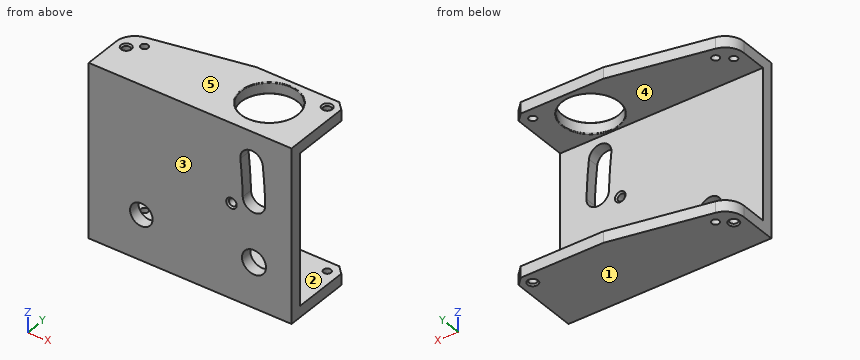
from build123d import *

# Parameters (mm, degrees)
SKETCH1_W      = 27
SKETCH1_H      = 23
SKETCH1_R      = 1.6
SKETCH1_R_2    = 1.5
SKETCH1_R_3    = 0.5
EXTRUDE1_DEPTH = 1.5
SKETCH2_R      = 0.5
SKETCH2_R_2    = 3.75
EXTRUDE2_DEPTH = 1.5
SKETCH3_R      = 0.5
EXTRUDE3_DEPTH = 1.5
FILLET1_R      = 0.1
CHAMFER1_SIZE  = 0.2
FILLET2_R      = 2.5


with BuildPart() as part:
    # Sketch1 → Extrude1 (new body)
    with BuildSketch(Plane(origin=(0, 0, 0), x_dir=(1, 0, 0), z_dir=(0, 1, 0))):
        with Locations((-8.5, -5.5)):
            Rectangle(SKETCH1_W, SKETCH1_H)
        with Locations(Location((0, 0, 0), (0, 0, 270))):  # turned: the seam where the file's is
            Circle(SKETCH1_R, mode=Mode.SUBTRACT)
        with Locations(Location((-15, 0, 0), (0, 0, 270))):  # turned: the seam where the file's is
            Circle(SKETCH1_R_2, mode=Mode.SUBTRACT)
        with Locations(Location((-3, -6.5, 0), (0, 0, 270))):  # turned: the seam where the file's is
            Circle(SKETCH1_R_3, mode=Mode.SUBTRACT)
        with BuildLine():
            ThreePointArc((-1.814657257, -12.850061187), (-1.613249333, -10.406431255), (-1.49938813, -7.957160339))
            ThreePointArc((-1.49938813, -7.957160339), (0.042839661, -6.50061187), (1.49938813, -8.042839661))
            ThreePointArc((1.49938813, -8.042839661), (1.380542383, -10.599333203), (1.170317351, -13.149938813))
            ThreePointArc((1.170317351, -13.149938813), (-0.472108766, -14.492487304), (-1.814657257, -12.850061187))
        make_face(mode=Mode.SUBTRACT)
    extrude(amount=EXTRUDE1_DEPTH)

    # Sketch2 → Extrude2 (add)
    with BuildSketch(Plane.XY.offset(17)):
        Polygon((-22, 1.5), (5, 1.5), (5, 9), (4, 10), (-7, 10), (-22, 7), align=None)
        with Locations((3.5, 8.5)):
            Circle(SKETCH2_R, mode=Mode.SUBTRACT)
        with Locations((-2, 5.5)):
            Circle(SKETCH2_R_2, mode=Mode.SUBTRACT)
        with Locations((-20.5, 4.75)):
            Circle(SKETCH2_R, mode=Mode.SUBTRACT)
        with Locations((-19, 6)):
            Circle(SKETCH2_R, mode=Mode.SUBTRACT)
    extrude(amount=-EXTRUDE2_DEPTH)

    # Sketch3 → Extrude3 (add)
    with BuildSketch(Plane(origin=(0, 0, -6), x_dir=(-1, 0, 0), z_dir=(0, 0, -1))):
        Polygon((-5, 1.5), (22, 1.5), (22, 7), (7, 10), (-4, 10), (-5, 9), align=None)
        with Locations(Location((-3.5, 8.5, 0), (0, 0, 180))):  # turned: the seam where the file's is
            Circle(SKETCH3_R, mode=Mode.SUBTRACT)
        with Locations(Location((20.5, 4.75, 0), (0, 0, 180))):  # turned: the seam where the file's is
            Circle(SKETCH3_R, mode=Mode.SUBTRACT)
        with Locations(Location((19, 6, 0), (0, 0, 180))):  # turned: the seam where the file's is
            Circle(SKETCH3_R, mode=Mode.SUBTRACT)
    extrude(amount=-EXTRUDE3_DEPTH)

    # Fillet1
    fillet1_edges = [part.edges().sort_by_distance(p)[0] for p in [
        (-5.75, 5.5, 15.5),
        (-5.75, 5.5, 17),
    ]]
    fillet(fillet1_edges, radius=FILLET1_R)

    # Chamfer1
    chamfer1_edges = [part.edges().sort_by_distance(p)[0] for p in [
        (-3, 0, 6),
        (-3, 1.5, 6),
        (3, 8.5, 17),
        (-21, 4.75, 17),
        (3, 8.5, -6),
        (-21, 4.75, -6),
    ]]
    chamfer(chamfer1_edges, length=CHAMFER1_SIZE)

    # Fillet2
    fillet2_edges = [part.edges().sort_by_distance(p)[0] for p in [
        (-22, 7, 16.25),
        (-22, 7, -5.25),
    ]]
    fillet(fillet2_edges, radius=FILLET2_R)


solid = part.part
Read the model definition and answer for the solid it produces. Units are mm, in the model's axes. Face numbers are marked on the shaded views. A direction names the side the tool comes from. Round coordinates to 2 decimals unless told otherwise and drop trailing zeros. Order: outer loops, then holes, each group sorted by start corner. A loop starts at its lowest first (then second) coordinate and runs counter-clockwise, first axis right, second up. Notation, with made-up numbers: (67.5, 12.25) - (104.5, 12.25) arc R29 ccw to (104.5, 47.25) - close; hole circle Ø6 at (48.5, 6.25). An arc over 180 degrees is marked (long way). Use one line per item in the form item = value. Start each with the question number.
(1) The part is cut by section D-D (x = 0). Count the separate pieces of the cut face and the enclosed holes in it, then the cut area to 3 significant figures.
(2) The part is cut by section C-C (z = 4). Give the vertices of the cut face in (x, y), then the cut area to 3 significant figures.
(3) The part is cut by section A-A (x = -19). Give the vertices of the cut face in (y, z).
(4) The part is cut by section B-B (z = 9). Give the vertices of the cut face in (x, y).
(5) Determine the mould class of the marked faces 3, 4 and 5 for opening direction Z: +Z half, -Z half, draft (parallel to the pull), parting line (faces both ways), or undercut.
(6) For the marked faces 1 and 2, determine the directions among +Z, -Z, +X, -X, +Y, -Y from which every point of the face is accessible in a straight line to the end or side of a thin tool.
(7) Find the intervals of material crossed by line 1 along Z through (x, y) = (-7.25, 3); line 2 along X through (y, z) = (0.9, 0); line 3 along Y through (x, z) = (-18.75, 12.25), in increasing order. Write a range as from..to.
(8) Flat-ended cylindrical pins translate along their axes: pin 1 Ø8 at (x, z) = (-9, -1) entering from +Y; pin 2 Ø1.5 at (x, z) = (-8, 3) entering from +Y; pin 3 Ø4.5 at (x, y) = (-2, 5.5) entering from +Z. Find the tip coordinate at first contact, or state that the pin passes through.
Checked values:
q1.separate_pieces = 4
q1.enclosed_holes = 0
q1.area = 33.7 mm^2
q2.outline = (-22, 0) - (5, 0) - (5, 1.5) - (-22, 1.5) - close
q2.area = 40.5 mm^2
q3.outline = (0, -6) - (5.5, -6) - (5.5, -4.5) - (1.5, -4.5) - (1.5, 15.5) - (5.5, 15.5) - (5.5, 17) - (0, 17) - close; (6.5, -6) - (7.6, -6) - (7.6, -4.5) - (6.5, -4.5) - close; (6.5, 15.5) - (7.6, 15.5) - (7.6, 17) - (6.5, 17) - close
q4.outline = (-22, 0) - (-1.54, 0) - (-1.54, 1.5) - (-22, 1.5) - close; (1.47, 0) - (5, 0) - (5, 1.5) - (1.47, 1.5) - close
q5.face_3 = draft
q5.face_4 = undercut
q5.face_5 = +Z half
q6.face_1 = -Z, +X, -X, +Y, -Y
q6.face_2 = +X, -X, +Y
q7.line_1 = -6..-4.5, 15.5..17
q7.line_2 = -22..-16.5, -13.5..-1.6, 1.6..5
q7.line_3 = 0..1.5
q8.pin_1 = 9.99
q8.pin_2 = 1.5
q8.pin_3 = -4.5
